Could you check a few things on this model? Use its own coordinates, in mm. Round coordinates to 2 decimals unless told otherwise and drop trailing zeros. Loops run counter-clockwise (first coordinate to the right, second up) from the corner with the lowest first, then second, coordinate; pieces in that order, holes last. Notation, with made-up numbers: (68.5, 69) - (73.5, 69) arc R28 ccw to (73.5, 101) - close; hole circle Ø3 at (83.25, -11). An arc over 180 degrees is marked (long way). Use one line per item in the form item = value.
```python
from build123d import *
from OCP.BRepFilletAPI import BRepFilletAPI_MakeChamfer

# Parameters (mm, degrees)
BOSS_EXTRUDE1_DEPTH = 6
SKETCH2_W           = 6.35
SKETCH2_H           = 69.85
SKETCH2_W_2         = 7.62
SKETCH2_H_2         = 5.08
SKETCH2_W_3         = 5.08
SKETCH2_H_3         = 7.62
BOSS_EXTRUDE2_DEPTH = 6
FILLET1_R           = 1.27
SKETCH3_W           = 6
SKETCH3_H           = 19.05
CUT_EXTRUDE1_DEPTH  = 275.000314781
FILLET2_R           = 2.54
SKETCH4_W           = 7.112
SKETCH4_H           = 10.795
SKETCH4_W_2         = 3.175
SKETCH4_H_2         = 3.556
CUT_EXTRUDE2_DEPTH  = 275.000314781
FILLET3_R           = 1.27
SKETCH5_R           = 1.524
SKETCH5_W           = 6.35
SKETCH5_H           = 22.86
CUT_EXTRUDE3_DEPTH  = 275.000314781
SKETCH6_W           = 7.3152
SKETCH6_H           = 2.9972
SKETCH6_W_2         = 2.9972
SKETCH6_H_2         = 7.3152
SKETCH6_W_3         = 6.858
SKETCH6_W_4         = 4.7625
SKETCH6_H_3         = 15.24
SKETCH6_W_5         = 15.24
SKETCH6_H_4         = 4.7625
CUT_EXTRUDE4_DEPTH  = 275.000314781
FILLET4_R           = 0.762
CHAMFER1_SIZE       = 0.381
CHAMFER1_SIZE2      = 1.046788897
CHAMFER2_SIZE       = 0.381
CHAMFER2_SIZE2      = 1.046788897


with BuildPart() as part:
    # Sketch1 → Boss-Extrude1 (new body)
    with BuildSketch(Plane.XY):
        Polygon((0, 0), (190.5, 0), (190.5, 44.45), (38.1, 44.45), (38.1, 196.85), (0, 196.85), align=None)
    extrude(amount=BOSS_EXTRUDE1_DEPTH)

    # Sketch2 → Boss-Extrude2 (add)
    with BuildSketch(Plane.XY.offset(6)):
        Polygon((0, 177.8), (-6.35, 177.8), (-6.35, 180.975), (-10.16, 180.975), (-10.16, 171.45), (0, 171.45), align=None)
        with Locations((-3.175, 34.925)):
            Rectangle(SKETCH2_W, SKETCH2_H)
        Polygon((0, 107.95), (-6.35, 107.95), (-6.35, 111.125), (-10.16, 111.125), (-10.16, 101.6), (0, 101.6), align=None)
        with Locations((72.39, 46.99)):
            Rectangle(SKETCH2_W_2, SKETCH2_H_2)
        with Locations((186.69, 46.99)):
            Rectangle(SKETCH2_W_2, SKETCH2_H_2)
        with Locations((40.64, 193.04)):
            Rectangle(SKETCH2_W_3, SKETCH2_H_3)
        with Locations((40.64, 104.14)):
            Rectangle(SKETCH2_W_3, SKETCH2_H_3)
    extrude(amount=-BOSS_EXTRUDE2_DEPTH)

    # Fillet1
    fillet1_edges = [part.edges().sort_by_distance(p)[0] for p in [
        (-10.16, 171.45, 3),
        (-10.16, 180.975, 3),
        (-6.35, 180.975, 3),
        (-10.16, 101.6, 3),
        (-10.16, 111.125, 3),
        (-6.35, 111.125, 3),
    ]]
    fillet(fillet1_edges, radius=FILLET1_R)

    # Sketch3 → Cut-Extrude1 (cut, through all)
    with BuildSketch(Plane.XY.offset(6)):
        with Locations((187.5, 9.525)):
            Rectangle(SKETCH3_W, SKETCH3_H)
    extrude(amount=-CUT_EXTRUDE1_DEPTH, mode=Mode.SUBTRACT)

    # Fillet2
    fillet2_edges = [part.edges().sort_by_distance(p)[0] for p in [
        (-6.35, 0, 3),
    ]]
    fillet(fillet2_edges, radius=FILLET2_R)

    # Sketch4 → Cut-Extrude2 (cut, through all)
    with BuildSketch(Plane.XY.offset(6)):
        with Locations((9.556, 178.054)):
            Rectangle(SKETCH4_W, SKETCH4_H)
        with Locations((1.5875, 146.05)):
            Rectangle(SKETCH4_W_2, SKETCH4_H_2)
    extrude(amount=-CUT_EXTRUDE2_DEPTH, mode=Mode.SUBTRACT)

    # Fillet3
    fillet3_edges = [part.edges().sort_by_distance(p)[0] for p in [
        (13.112, 183.4515, 3),
        (13.112, 172.6565, 3),
        (6, 172.6565, 3),
        (6, 183.4515, 3),
    ]]
    fillet(fillet3_edges, radius=FILLET3_R)

    # Sketch5 → Cut-Extrude3 (cut, through all)
    with BuildSketch(Plane.XY.offset(6)):
        with Locations((10.7442, 124.206)):
            Circle(SKETCH5_R)
        with Locations((10.7442, 86.106)):
            Circle(SKETCH5_R)
        with Locations((10.7442, 105.156)):
            Rectangle(SKETCH5_W, SKETCH5_H)
    extrude(amount=-CUT_EXTRUDE3_DEPTH, mode=Mode.SUBTRACT)

    # Sketch6 → Cut-Extrude4 (cut, through all)
    with BuildSketch(Plane.XY.offset(6)):
        with Locations((34.4424, 181.3814)):
            Rectangle(SKETCH6_W, SKETCH6_H)
        with Locations((34.4424, 92.4814)):
            Rectangle(SKETCH6_W, SKETCH6_H)
        with Locations((84.0486, 40.7924)):
            Rectangle(SKETCH6_W_2, SKETCH6_H_2)
        with Locations((175.0314, 40.7924)):
            Rectangle(SKETCH6_W_2, SKETCH6_H_2)
        with Locations((181.071, 9.525)):
            Rectangle(SKETCH6_W_3, SKETCH6_H)
        with Locations((35.71875, 148.87448)):
            Rectangle(SKETCH6_W_4, SKETCH6_H_3)
        with Locations((104.75976, 42.06875)):
            Rectangle(SKETCH6_W_5, SKETCH6_H_4)
    extrude(amount=-CUT_EXTRUDE4_DEPTH, mode=Mode.SUBTRACT)

    # Fillet4
    fillet4_edges = [part.edges().sort_by_distance(p)[0] for p in [
        (7.5692, 93.726, 3),
        (7.5692, 116.586, 3),
        (13.9192, 116.586, 3),
        (13.9192, 93.726, 3),
        (33.3375, 141.25448, 3),
        (33.3375, 156.49448, 3),
        (97.13976, 39.6875, 3),
        (112.37976, 39.6875, 3),
    ]]
    fillet(fillet4_edges, radius=FILLET4_R)

    # Chamfer1: one chamfer whose edges measure the first distance from different faces: ONE call of the kernel's chamfer builder (chamfer() names one face for all edges)
    chamfer1_edges_1 = [part.edges().sort_by_distance(p)[0] for p in [
        (38.1, 182.88, 3),
    ]]
    chamfer1_side_1 = [part.faces().sort_by_distance(p)[0] for p in [
        (38.1, 186.055, 3),
    ]]
    chamfer1_edges_2 = [part.edges().sort_by_distance(p)[0] for p in [
        (38.1, 179.8828, 3),
    ]]
    chamfer1_side_2 = [part.faces().sort_by_distance(p)[0] for p in [
        (38.1, 168.18864, 3),
    ]]
    chamfer1_edges_3 = [part.edges().sort_by_distance(p)[0] for p in [
        (38.1, 93.98, 3),
    ]]
    chamfer1_side_3 = [part.faces().sort_by_distance(p)[0] for p in [
        (38.1, 97.155, 3),
    ]]
    chamfer1_edges_4 = [part.edges().sort_by_distance(p)[0] for p in [
        (38.1, 90.9828, 3),
    ]]
    chamfer1_side_4 = [part.faces().sort_by_distance(p)[0] for p in [
        (38.1, 67.7164, 3),
    ]]
    chamfer1_edges_5 = [part.edges().sort_by_distance(p)[0] for p in [
        (82.55, 44.45, 3),
    ]]
    chamfer1_side_5 = [part.faces().sort_by_distance(p)[0] for p in [
        (79.375, 44.45, 3),
    ]]
    chamfer1_edges_6 = [part.edges().sort_by_distance(p)[0] for p in [
        (85.5472, 44.45, 3),
    ]]
    chamfer1_side_6 = [part.faces().sort_by_distance(p)[0] for p in [
        (91.34348, 44.45, 3),
    ]]
    chamfer1_edges_7 = [part.edges().sort_by_distance(p)[0] for p in [
        (173.5328, 44.45, 3),
    ]]
    chamfer1_side_7 = [part.faces().sort_by_distance(p)[0] for p in [
        (142.95628, 44.45, 3),
    ]]
    chamfer1_edges_8 = [part.edges().sort_by_distance(p)[0] for p in [
        (176.53, 44.45, 3),
    ]]
    chamfer1_side_8 = [part.faces().sort_by_distance(p)[0] for p in [
        (179.705, 44.45, 3),
    ]]
    chamfer1_edges_9 = [part.edges().sort_by_distance(p)[0] for p in [
        (184.5, 11.0236, 3),
    ]]
    chamfer1_side_9 = [part.faces().sort_by_distance(p)[0] for p in [
        (184.5, 15.0368, 3),
    ]]
    chamfer1_edges_10 = [part.edges().sort_by_distance(p)[0] for p in [
        (184.5, 8.0264, 3),
    ]]
    chamfer1_side_10 = [part.faces().sort_by_distance(p)[0] for p in [
        (184.5, 4.0132, 3),
    ]]
    chamfer1 = BRepFilletAPI_MakeChamfer(part.part.solid().wrapped)
    for e in chamfer1_edges_1:
        chamfer1.Add(CHAMFER1_SIZE, CHAMFER1_SIZE2, e.wrapped, chamfer1_side_1[0].wrapped)  # the first distance lies on this face
    for e in chamfer1_edges_2:
        chamfer1.Add(CHAMFER1_SIZE, CHAMFER1_SIZE2, e.wrapped, chamfer1_side_2[0].wrapped)  # the first distance lies on this face
    for e in chamfer1_edges_3:
        chamfer1.Add(CHAMFER1_SIZE, CHAMFER1_SIZE2, e.wrapped, chamfer1_side_3[0].wrapped)  # the first distance lies on this face
    for e in chamfer1_edges_4:
        chamfer1.Add(CHAMFER1_SIZE, CHAMFER1_SIZE2, e.wrapped, chamfer1_side_4[0].wrapped)  # the first distance lies on this face
    for e in chamfer1_edges_5:
        chamfer1.Add(CHAMFER1_SIZE, CHAMFER1_SIZE2, e.wrapped, chamfer1_side_5[0].wrapped)  # the first distance lies on this face
    for e in chamfer1_edges_6:
        chamfer1.Add(CHAMFER1_SIZE, CHAMFER1_SIZE2, e.wrapped, chamfer1_side_6[0].wrapped)  # the first distance lies on this face
    for e in chamfer1_edges_7:
        chamfer1.Add(CHAMFER1_SIZE, CHAMFER1_SIZE2, e.wrapped, chamfer1_side_7[0].wrapped)  # the first distance lies on this face
    for e in chamfer1_edges_8:
        chamfer1.Add(CHAMFER1_SIZE, CHAMFER1_SIZE2, e.wrapped, chamfer1_side_8[0].wrapped)  # the first distance lies on this face
    for e in chamfer1_edges_9:
        chamfer1.Add(CHAMFER1_SIZE, CHAMFER1_SIZE2, e.wrapped, chamfer1_side_9[0].wrapped)  # the first distance lies on this face
    for e in chamfer1_edges_10:
        chamfer1.Add(CHAMFER1_SIZE, CHAMFER1_SIZE2, e.wrapped, chamfer1_side_10[0].wrapped)  # the first distance lies on this face
    add(Compound.cast(chamfer1.Shape()), mode=Mode.REPLACE)

    # Chamfer2: one chamfer whose edges measure the first distance from different faces: ONE call of the kernel's chamfer builder (chamfer() names one face for all edges)
    chamfer2_edges_1 = [part.edges().sort_by_distance(p)[0] for p in [
        (68.58, 49.53, 3),
        (76.2, 49.53, 3),
    ]]
    chamfer2_side_1 = [part.faces().sort_by_distance(p)[0] for p in [
        (72.39, 49.53, 3),
    ]]
    chamfer2_edges_2 = [part.edges().sort_by_distance(p)[0] for p in [
        (190.5, 49.53, 3),
        (182.88, 49.53, 3),
    ]]
    chamfer2_side_2 = [part.faces().sort_by_distance(p)[0] for p in [
        (186.69, 49.53, 3),
    ]]
    chamfer2_edges_3 = [part.edges().sort_by_distance(p)[0] for p in [
        (43.18, 196.85, 3),
        (43.18, 189.23, 3),
    ]]
    chamfer2_side_3 = [part.faces().sort_by_distance(p)[0] for p in [
        (43.18, 193.04, 3),
    ]]
    chamfer2_edges_4 = [part.edges().sort_by_distance(p)[0] for p in [
        (43.18, 107.95, 3),
        (43.18, 100.33, 3),
    ]]
    chamfer2_side_4 = [part.faces().sort_by_distance(p)[0] for p in [
        (43.18, 104.14, 3),
    ]]
    chamfer2 = BRepFilletAPI_MakeChamfer(part.part.solid().wrapped)
    for e in chamfer2_edges_1:
        chamfer2.Add(CHAMFER2_SIZE, CHAMFER2_SIZE2, e.wrapped, chamfer2_side_1[0].wrapped)  # the first distance lies on this face
    for e in chamfer2_edges_2:
        chamfer2.Add(CHAMFER2_SIZE, CHAMFER2_SIZE2, e.wrapped, chamfer2_side_2[0].wrapped)  # the first distance lies on this face
    for e in chamfer2_edges_3:
        chamfer2.Add(CHAMFER2_SIZE, CHAMFER2_SIZE2, e.wrapped, chamfer2_side_3[0].wrapped)  # the first distance lies on this face
    for e in chamfer2_edges_4:
        chamfer2.Add(CHAMFER2_SIZE, CHAMFER2_SIZE2, e.wrapped, chamfer2_side_4[0].wrapped)  # the first distance lies on this face
    add(Compound.cast(chamfer2.Shape()), mode=Mode.REPLACE)


solid = part.part
```
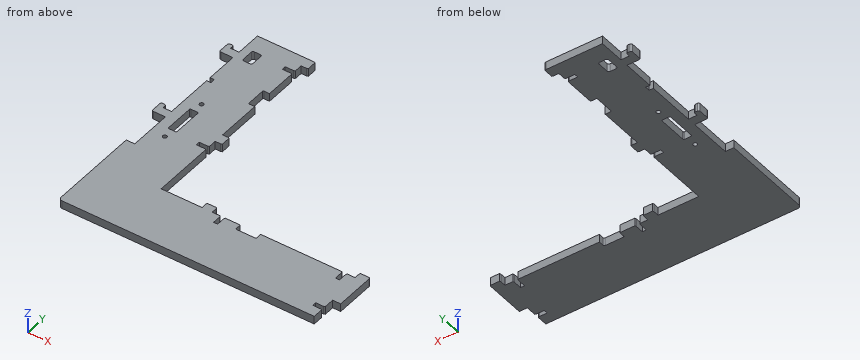
1. If we section it at A-A, the plane y = 166: Write out the boundary of the cut face in (x, z), plus the area to 3 significant figures.
Solution:
outline = (0, 0) - (38.1, 0) - (38.1, 6) - (0, 6) - close
area = 229 mm^2
2. If we section it at B-B, the plane x = 71.5: Write out the boundary of the cut face in (y, z), plus the area to 3 significant figures.
Solution:
outline = (0, 0) - (49.53, 0) - (49.53, 6) - (0, 6) - close
area = 297 mm^2
3. Please list where these lines run through material, in increasing order: line 1 along Y through (x, z) = (-1, 4.75); line 2 along X through (y, z) = (45.5, 1.3); line 3 along Y through (x, z) = (2.5, 2.3).
Solution:
line_1 = 0 to 69.85, 101.6 to 107.95, 171.45 to 177.8
line_2 = -6.35 to 38.1, 68.58 to 76.2, 182.88 to 190.5
line_3 = 0 to 144.27, 147.83 to 196.85
4. If we section it at C-C, the plane z = 4: Count the separate pieces of the cut face and the enclosed holes in it, plus the area to 3 significant figures.
Solution:
separate_pieces = 1
enclosed_holes = 4
area = 14,400 mm^2
5. For P1, Ø3.5, axis at y = 92, z = 2.5, coming from the +X side; P2, Ø3, axis at x = 59.5, z = 4, coming from the +Y side; P3, Ø1.5, axis at x = 174.5, z = 4.5, coming from the +Y side, each with a flat end and sliding along its axis, tell me the tip position at first contact or that it passes through.
Solution:
P1 = 38.1
P2 = 44.45
P3 = 37.13
